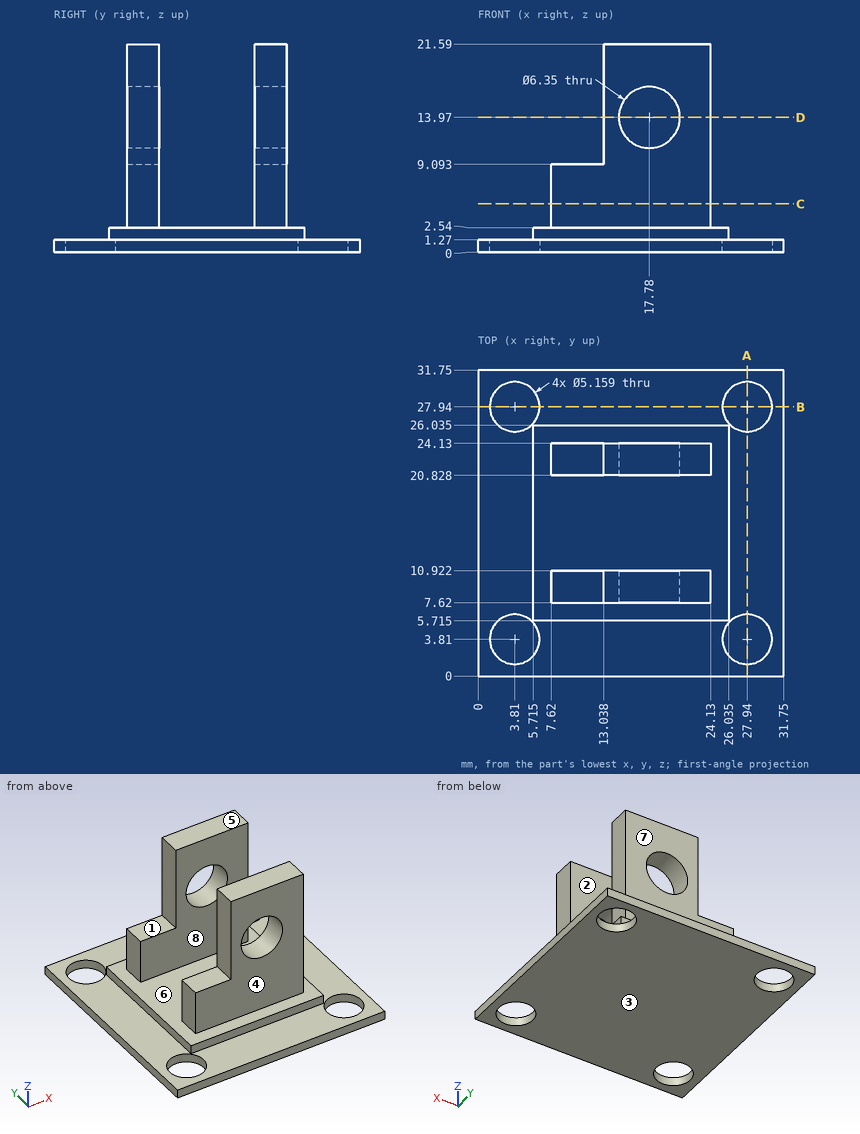
Here's the drawing with two shaded views (mm, measured from the low corner). I have some questions. A direction names the side the tool comes from. Coordinates: 2 decimals unless noted, no trailing zeros. Write each loop counter-clockwise with the first axis right and the second up, starting at its lowest first coordinate (ties: lowest second). Pieces come first, ordered by that corner, then holes. Notation, with made-up numbers: (19, 11) -> (63, 11) arc R32 cw to (63, 49) -> close; hole circle Ø7 at (43, 85.25). An arc over 180 degrees is marked (long way). Use a Markdown table: item, result. Add a question column.
(1) For the marked faces 1, 2, 3 and 4, which set-ups out of +Z, -Z, +X, -X, +Y, -Y let a thin tool reach every point of the face, with its end or its side?
(2) Please list where these lines run through material, in increasing order: line 1 (Y direction, x = 19.5, z = 20.75); line 2 (Y direction, x = 3.81, z = 0.4); line 3 (Z direction, x = 17.78, y = 21.5) (1 decimal).
(3) I'm going to push flat-ended pins straight in: P1, Ø1.7, axis at x = 10.5, y = 21.5, coming from the +Z side; P2, Ø2.5, axis at y = 10, z = 17.5, coming from the -X side; P3, Ø1.5, axis at y = 10.5, z = 9.5, coming from the +X side. Where does each tip first touch, or does it pass through?
(4) If we section it at C-C, the plane z = 5: Write out the boundary of the cut face in (x, y), and give its area (3 significant figures).
(5) We'd pull the mould along Y, two halves only. Please class the marked faces 5, 6, 7 and 8: +Y half, -Y half, draft (parallel to the pull), parting line (faces both ways), or undercut.
(6) If we section it at A-A, the plane x = 27.94: Write out the boundary of the cut face in (y, z).
(7) If we section it at D-D, the plane z = 13.97: Write out the boundary of the cut face in (x, y) (1 decimal).
Outcome:
| question | item | result |
|---|---|---|
| 1 | face 1 | +Z, -X, +Y, -Y |
| 1 | face 2 | +Z, +X, -X |
| 1 | face 3 | -Z, +X, -X, +Y, -Y |
| 1 | face 4 | +Z, +X, -X, -Y |
| 2 | line 1 | y = 7.62 to 10.92, 20.83 to 24.13 |
| 2 | line 2 | y = 0 to 1.23, 6.39 to 25.36, 30.52 to 31.75 |
| 2 | line 3 | z = 0 to 10.8, 17.1 to 21.6 |
| 3 | P1 | stops at z = 9.09 |
| 3 | P2 | stops at x = 13.04 |
| 3 | P3 | stops at x = 24.13 |
| 4 | outline | (7.62, 7.62) -> (24.13, 7.62) -> (24.13, 10.92) -> (7.62, 10.92) -> close; (7.62, 20.83) -> (24.13, 20.83) -> (24.13, 24.13) -> (7.62, 24.13) -> close |
| 4 | area | 109 mm^2 |
| 5 | face 5 | draft |
| 5 | face 6 | undercut |
| 5 | face 7 | +Y half |
| 5 | face 8 | undercut |
| 6 | outline | (0, 0) -> (1.23, 0) -> (1.23, 1.27) -> (0, 1.27) -> close; (6.39, 0) -> (25.36, 0) -> (25.36, 1.27) -> (6.39, 1.27) -> close; (30.52, 0) -> (31.75, 0) -> (31.75, 1.27) -> (30.52, 1.27) -> close |
| 7 | outline | (13, 7.6) -> (14.6, 7.6) -> (14.6, 10.9) -> (13, 10.9) -> close; (13, 20.8) -> (14.6, 20.8) -> (14.6, 24.1) -> (13, 24.1) -> close; (21, 7.6) -> (24.1, 7.6) -> (24.1, 10.9) -> (21, 10.9) -> close; (21, 20.8) -> (24.1, 20.8) -> (24.1, 24.1) -> (21, 24.1) -> close |
